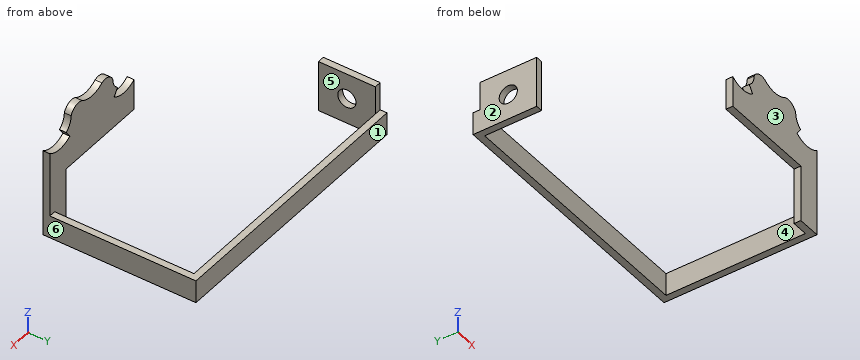
from build123d import *

# Parameters (mm, degrees)
BOSS_EXTRUDE1_DEPTH = 3
SKETCH3_W           = 10
SKETCH3_H           = 3
BOSS_EXTRUDE2_DEPTH = 25
SKETCH5_W           = 3
SKETCH5_H           = 10
BOSS_EXTRUDE4_DEPTH = 64.25
SKETCH7_W           = 10
SKETCH7_H           = 3
BOSS_EXTRUDE5_DEPTH = 115.21
SKETCH8_W           = 3
SKETCH8_H           = 22.5
BOSS_EXTRUDE6_DEPTH = 25
SKETCH10_R          = 4
CUT_EXTRUDE1_DEPTH  = 3


with BuildPart() as part:
    # Sketch2 → Boss-Extrude1 (new body)
    with BuildSketch(Plane(origin=(0, 0, 0), x_dir=(1, 0, 0), z_dir=(0, 1, 0))):
        with BuildLine():
            Line((-15.860247962, 17.20906431), (-13.694996915, 20.301363277))
            ThreePointArc((-13.694996915, 20.301363277), (-19.875283017, 22.25), (-26.055569119, 20.301363277))
            Line((-26.055569119, 20.301363277), (-26.055569119, 33.889213566))
            Line((-26.055569119, 33.889213566), (26.055569119, 33.889213566))
            Line((26.055569119, 33.889213566), (26.055569119, 20.301363277))
            ThreePointArc((26.055569119, 20.301363277), (19.875283017, 22.25), (13.694996915, 20.301363277))
            Line((13.694996915, 20.301363277), (15.860247962, 17.20906431))
            ThreePointArc((15.860247962, 17.20906431), (13.666207185, 14.707240293), (12.875283017, 11.475))
            ThreePointArc((12.875283017, 11.475), (10.090653959, 8.727908609), (6.180286102, 8.826363277))
            ThreePointArc((6.180286102, 8.826363277), (0, 10.775), (-6.180286102, 8.826363277))
            ThreePointArc((-6.180286102, 8.826363277), (-10.090653959, 8.727908609), (-12.875283017, 11.475))
            ThreePointArc((-12.875283017, 11.475), (-13.666207185, 14.707240293), (-15.860247962, 17.20906431))
        make_face()
    extrude(amount=BOSS_EXTRUDE1_DEPTH)

    # Sketch3 → Boss-Extrude2 (add)
    with BuildSketch(Plane(origin=(0, 0, -33.889213566), x_dir=(-1, 0, 0), z_dir=(0, 0, -1))):
        with Locations((-21.055569119, 1.5)):
            Rectangle(SKETCH3_W, SKETCH3_H)
    extrude(amount=BOSS_EXTRUDE2_DEPTH)

    # Sketch5 → Boss-Extrude4 (add)
    with BuildSketch(Plane(origin=(0, 3, 0), x_dir=(1, 0, 0), z_dir=(0, 1, 0))):
        with Locations((24.555569119, 53.889213566)):
            Rectangle(SKETCH5_W, SKETCH5_H)
    extrude(amount=BOSS_EXTRUDE4_DEPTH)

    # Sketch7 → Boss-Extrude5 (add)
    with BuildSketch(Plane.ZY.offset(-23.055569119)):
        with Locations((-53.889213566, 65.75)):
            Rectangle(SKETCH7_W, SKETCH7_H)
    extrude(amount=BOSS_EXTRUDE5_DEPTH)

    # Sketch8 → Boss-Extrude6 (add)
    with BuildSketch(Plane.XZ.offset(-64.25)):
        with Locations((-90.654430881, -47.639213566)):
            Rectangle(SKETCH8_W, SKETCH8_H)
    extrude(amount=BOSS_EXTRUDE6_DEPTH)

    # Sketch10 → Cut-Extrude1 (cut)
    with BuildSketch(Plane.ZY.offset(92.154430881)):
        with Locations((-47.639213566, 51.75)):
            Circle(SKETCH10_R)
    extrude(amount=-CUT_EXTRUDE1_DEPTH, mode=Mode.SUBTRACT)


solid = part.part
Input: part model. Units: mm. Frame: model coordinates. Face numbers are marked on the shaded views. A direction names the side the tool comes from. Coordinates: 2 decimals unless noted, no trailing zeros. Order: outer loops, then holes, each group sorted by start corner. A loop starts at its lowest first (then second) coordinate and runs counter-clockwise, first axis right, second up. Notation, with made-up numbers: M 16,62 L 42,62 A20 ccw 42,78 Z; hole C 58.5,-1 d10. An arc over 180 degrees is marked long. Answer in a Markdown table with one row per item.
(1) Section query C-C, the plane x = 2. Output: boundary loops of the cut face in (y, z), plus the area to 3 significant figures.
Numbers:
| item | result |
|---|---|
| outline | M 0,-33.89 L 3,-33.89 L 3,-10.59 L 0,-10.59 Z; M 64.25,-58.89 L 67.25,-58.89 L 67.25,-48.89 L 64.25,-48.89 Z |
| area | 99.9 mm^2 |
(2) Access query for the marked faces 5 and 6. Directions: +Z, -Z, +X, -X, +Y, -Y. A direction counts if a zero-diameter tool reaches every point of the face in a straight line with its end or side. Return the directions, or none.
Numbers:
| item | result |
|---|---|
| face 5 | +Z, -Z, -Y |
| face 6 | +Z, -Z, +X, +Y, -Y |
(3) Section query B-B, the plane y = 41.5. Output: boundary loops of the cut face in (x, z).
Numbers:
| item | result |
|---|---|
| outline | M -92.15,-58.89 L -89.15,-58.89 L -89.15,-36.39 L -92.15,-36.39 Z; M 23.06,-58.89 L 26.06,-58.89 L 26.06,-48.89 L 23.06,-48.89 Z |
(4) Section query D-D, the plane x = -71. Output: boundary loops of the cut face in (y, z), plus the area to 3 significant figures.
Numbers:
| item | result |
|---|---|
| outline | M 64.25,-58.89 L 67.25,-58.89 L 67.25,-48.89 L 64.25,-48.89 Z |
| area | 30.0 mm^2 |
(5) Contact query for flat-ended pins moving along their axis: pin 1 Ø1.5 at (y, z) = (2, -25) entering from -X; pin 2 Ø1.5 at (x, y) = (-91, 51) entering from +Z; pin 3 Ø5 at (y, z) = (51.75, -47.64) entering from -X. Output: stop coordinate, or through.
Numbers:
| item | result |
|---|---|
| pin 1 | stops at x = -26.06 |
| pin 2 | stops at z = -36.39 |
| pin 3 | stops at x = 23.06 |
(6) Section query A-A, the plane y = 51.75. Output: boundary loops of the cut face in (x, z), plus the area to 3 significant figures.
Numbers:
| item | result |
|---|---|
| outline | M -92.15,-58.89 L -89.15,-58.89 L -89.15,-51.64 L -92.15,-51.64 Z; M -92.15,-43.64 L -89.15,-43.64 L -89.15,-36.39 L -92.15,-36.39 Z; M 23.06,-58.89 L 26.06,-58.89 L 26.06,-48.89 L 23.06,-48.89 Z |
| area | 73.5 mm^2 |
(7) Draft query along Y for the marked faces 1, 2, 3 and 4. Return one class per face: pulls with the +Y half, pulls with the -Y half, needs draft (parallel to the pull), parting line crosses it, or undercut.
Numbers:
| item | result |
|---|---|
| face 1 | pulls with the +Y half |
| face 2 | needs draft |
| face 3 | pulls with the -Y half |
| face 4 | undercut |
(8) Material intervals for line 1 (Y direction, x = -66, z = -53); line 2 (X direction, y = 12.5, z = -52); line 3 (Z direction, x = -91, y = 51), sorted ascending. Write a range as [from, to].
Numbers:
| item | result |
|---|---|
| line 1 | y = [64.25, 67.25] |
| line 2 | x = [23.06, 26.06] |
| line 3 | z = [-58.89, -51.57], [-43.71, -36.39] |
